The figure shows three views and two pictorial views of one solid part (mm, origin at its lowest corner). Answer the questions. A direction names the side the tool comes from. Coordinates: 2 decimals unless noted, no trailing zeros. Order: outer loops, then holes, each group sorted by start corner. A loop starts at its lowest first (then second) coordinate and runs counter-clockwise, first axis right, second up. Notation, with made-up numbers: M 79,-30 L 88,-30 A24 ccw 88,-8 Z; hole C 3,18.25 d8. An arc over 180 degrees is marked long. Answer in a Markdown table with one row per item. Add a question column.
Item 1: Flat-ended cylindrical pins translate along their axes: pin 1 Ø3 at (x, z) = (39.5, 3.5) entering from +Y; pin 2 Ø0.8 at (y, z) = (21, 4.5) entering from -X. Find the tip coordinate at first contact, or state that the pin passes through.
Item 2: Which of the six approach directions +Z, -Z, +X, -X, +Y, -Y give full straight-line access (tool end or side, diameter ignored) to the marked faces 1, 2 and 3?
Item 3: The part is cut by section A-A (z = 4.75). Write down the section's boundary in (x, y).
Item 4: Consider line 1 (Y direction, x = 36, z = 1); line 2 (X direction, y = 21.25, z = 3); line 3 (X direction, y = 19.5, z = 9.75). Determine where each line is inside the solid, lowest interval first. Write a range as from..to.
Item 5: The part is cut by section C-C (y = 18.5). Write down the section's boundary in (x, z).
Item 6: The part is cut by section B-B (x = 15). Write down the section's boundary in (y, z), then the cut area to 3 significant figures.
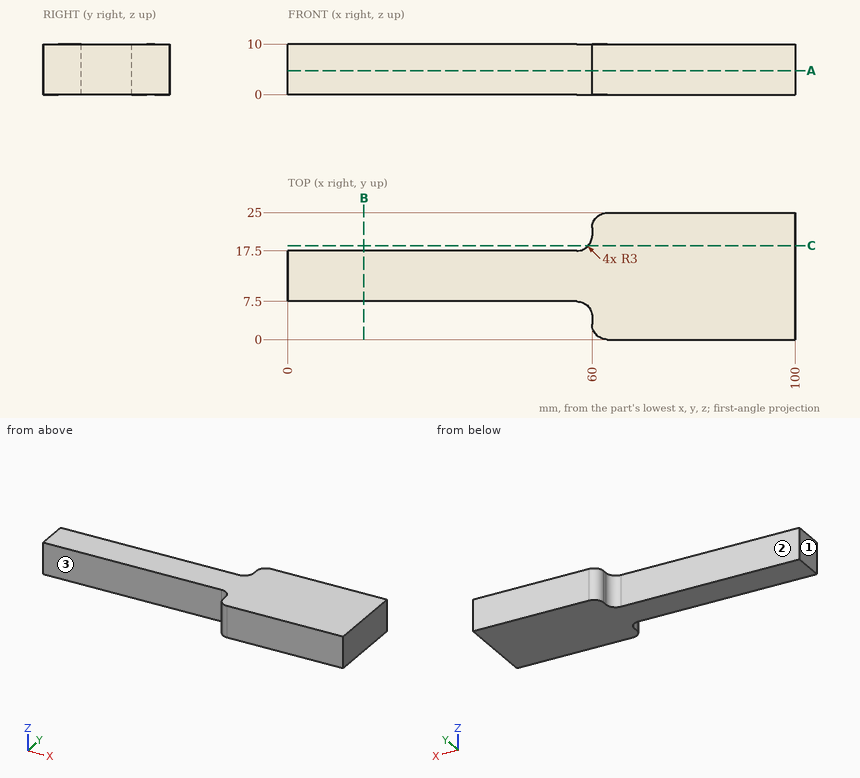
Reply:
| question | item | result |
|---|---|---|
| 1 | pin 1 | stops at y = 17.5 |
| 1 | pin 2 | stops at x = 60 |
| 2 | face 1 | +Z, -Z, -X, +Y, -Y |
| 2 | face 2 | +Z, -Z, -X, +Y |
| 2 | face 3 | +Z, -Z, -X, -Y |
| 3 | outline | M 0,7.5 L 57,7.5 A3 cw 60,4.5 L 60,3 A3 ccw 63,0 L 100,0 L 100,25 L 63,25 A3 ccw 60,22 L 60,20.5 A3 cw 57,17.5 L 0,17.5 Z |
| 4 | line 1 | y = 7.5..17.5 |
| 4 | line 2 | x = 60..100 |
| 4 | line 3 | x = 59.83..100 |
| 5 | outline | M 59.24,0 L 100,0 L 100,10 L 59.24,10 Z |
| 6 | outline | M 7.5,0 L 17.5,0 L 17.5,10 L 7.5,10 Z |
| 6 | area | 100 mm2 |
